```python
from build123d import *

# Parameters (mm, degrees)
BOSS_EXTRUDE1_DEPTH = 1
BOSS_EXTRUDE2_START = 0.5
BOSS_EXTRUDE2_DEPTH = 0.5
BOSS_EXTRUDE6_DEPTH = 0.5


with BuildPart() as part:
    # Sketch1 → Boss-Extrude1 (new, symmetric)
    with BuildSketch(Plane(origin=(0, 0, 0), x_dir=(0, 0, -1), z_dir=(1, 0, 0))):
        with BuildLine():
            Line((2.95, 0), (1.965, 7.729516129))
            ThreePointArc((1.965, 7.729516129), (0, 9.46), (-1.965, 7.729516129))
            Line((-1.965, 7.729516129), (-2.95, 0))
            Line((-2.95, 0), (-3.958086961, 0))
            Line((-3.958086961, 0), (-2.956977914, 7.855927438))
            ThreePointArc((-2.956977914, 7.855927438), (0, 10.46), (2.956977914, 7.855927438))
            Line((2.956977914, 7.855927438), (3.958086961, 0))
            Line((3.958086961, 0), (2.95, 0))
        make_face()
    extrude(amount=BOSS_EXTRUDE1_DEPTH, both=True)

    # Sketch2 → Boss-Extrude2 (add)
    with BuildSketch(Plane(origin=(1, 0, 0), x_dir=(0, 0, -1), z_dir=(1, 0, 0)).offset(BOSS_EXTRUDE2_START)):
        with BuildLine():
            Line((2.95, 0), (3.958086961, 0))
            Line((3.958086961, 0), (2.956977914, 7.855927438))
            ThreePointArc((2.956977914, 7.855927438), (0, 10.46), (-2.956977914, 7.855927438))
            Line((-2.956977914, 7.855927438), (-3.958086961, 0))
            Line((-3.958086961, 0), (-2.95, 0))
            Line((-2.95, 0), (2.95, 0))
        make_face()
    extrude(amount=-BOSS_EXTRUDE2_DEPTH)

    # Sketch3 → Boss-Extrude6 (add)
    with BuildSketch(Plane.ZY.offset(1)):
        with BuildLine():
            Line((-3.958086961, 0), (3.958086961, 0))
            Line((3.958086961, 0), (2.956977914, 7.855927438))
            ThreePointArc((2.956977914, 7.855927438), (0, 10.46), (-2.956977914, 7.855927438))
            Line((-2.956977914, 7.855927438), (-3.958086961, 0))
        make_face()
    extrude(amount=BOSS_EXTRUDE6_DEPTH)


solid = part.part
```
The listing builds one solid part. Answer for the finished solid, in the listing's coordinates (mm). A direction names the side the tool comes from. Give positions to 0.01 mm unless a question says otherwise; leave off trailing zeros. Order: outer loops, then holes, each group sorted by start corner. A loop starts at its lowest first (then second) coordinate and runs counter-clockwise, first axis right, second up. Notation, with made-up numbers: (53, 45.5) - (98, 45.5) arc R17 cw to (98, 66.5) - close; hole circle Ø7 at (-26, 52). An arc over 180 degrees is marked (long way). Use one line per item in the form item = value. Start each with the question number.
(1) A cutting plane is placed at A-A, the plane z = 0. Write down the section's boundary in (x, y).
(2) A cutting plane is placed at B-B, the plane y = 6. Write down the section's boundary in (x, z), then the cut area to 3 significant figures.
(3) A cutting plane is placed at D-D, the plane y = 7.5. Write down the section's boundary in (x, z).
(4) The mould has two halves that part along X. Classify faces 1 (the cylindrical face through (0.02, 10.46, 0.06)), 2 (the flat face through (1, 4, 0)), 3 (the flat face through (1.5, 4, 0)), 4 (the flat face through (-1.5, 4, 0)): released by +X, released by -X, zero draft, split by the parting line, or undercut.
(5) A flat-ended cylindrical pin translates along its axis: pin 1 Ø1 at (x, y) = (0, 5.5) entering from +Z. Find the tip coordinate at first contact, or state that the pin passes through.
(6) Consider line 1 (X direction, y = 2, z = 2); line 2 (Z direction, x = 0.6, y = 5.75); line 3 (Z direction, x = -0.7, y = 4.5). Determine where each line is inside the solid, lowest interval first. Write a range as from..to.
(7) For faces 5 (the flat face through (0.021, 3.873, 3.465)), 6 (the cylindrical face through (0.01, 9.46, -0.04)), determine the directions among +Z, -Z, +X, -X, +Y, -Y from which every point of the face is accessible in a straight line to the end or side of a thin tool.
(8) A cutting plane is placed at C-C, the plane x = -0.1. Write down the section's boundary in (y, z) (3 decimals).
Ans:
q1.outline = (-1.5, 0) - (-1, 0) - (-1, 9.46) - (1, 9.46) - (1, 0) - (1.5, 0) - (1.5, 10.46) - (-1.5, 10.46) - close
q2.outline = (-1.5, -3.19) - (1.5, -3.19) - (1.5, 3.19) - (-1.5, 3.19) - close; hole (-1, -2.19) - (1, -2.19) - (1, 2.19) - (-1, 2.19) - close
q2.area = 10.4 mm^2
q3.outline = (-1.5, -3) - (1.5, -3) - (1.5, 3) - (-1.5, 3) - close; hole (-1, -1.99) - (1, -1.99) - (1, 1.99) - (-1, 1.99) - close
q4.face_1 = zero draft
q4.face_2 = undercut
q4.face_3 = released by +X
q4.face_4 = released by -X
q5.pin_1 = 3.32
q6.line_1 = -1.5..-1, 1..1.5
q6.line_2 = -3.23..-2.22, 2.22..3.23
q6.line_3 = -3.38..-2.38, 2.38..3.38
q7.face_5 = +Z, +X, -X, +Y
q7.face_6 = -Y
q8.outline = (0, -3.958) - (7.856, -2.957) arc R2.981 ccw to (7.856, 2.957) - (0, 3.958) - (0, 2.95) - (7.73, 1.965) arc R1.981 cw to (7.73, -1.965) - (0, -2.95) - close
